Could you check a few things on this model? Use its own coordinates, in mm. Face numbers are marked on the shaded views. A direction names the side the tool comes from. Coordinates: 2 decimals unless noted, no trailing zeros.
```python
from build123d import *

# Parameters (mm, degrees)
SKETCH1_RX          = 12
SKETCH1_RY          = 6.5
SKETCH1_R           = 1.1
BOSS_EXTRUDE1_DEPTH = 1
SKETCH2_R           = 6.5
BOSS_EXTRUDE2_DEPTH = 2
SKETCH4_R           = 5.5
BOSS_EXTRUDE3_DEPTH = 7
BOSS_EXTRUDE5_START = 0.25
SKETCH7_R           = 5.5
BOSS_EXTRUDE5_DEPTH = 0.25
SKETCH5_R           = 0.75
CUT_EXTRUDE2_DEPTH  = 7
SKETCH6_R           = 0.75
BOSS_EXTRUDE4_DEPTH = 3.4
FILLET1_R           = 0.25


with BuildPart() as part:
    # Sketch1 → Boss-Extrude1 (new body)
    with BuildSketch(Plane(origin=(0, 0, 0), x_dir=(1, 0, 0), z_dir=(0, 1, 0))):
        with Locations(Location((0, 0), (0, 0, 180))):
            Ellipse(SKETCH1_RX, SKETCH1_RY)
        with Locations(Location((-9, 0, 0), (0, 0, 270))):
            Circle(SKETCH1_R, mode=Mode.SUBTRACT)
        with Locations(Location((9, 0, 0), (0, 0, 270))):
            Circle(SKETCH1_R, mode=Mode.SUBTRACT)
    extrude(amount=BOSS_EXTRUDE1_DEPTH)

    # Sketch2 → Boss-Extrude2 (add)
    with BuildSketch(Plane(origin=(0, 1, 0), x_dir=(1, 0, 0), z_dir=(0, 1, 0))):
        with Locations(Location((0, 0, 0), (0, 0, 270))):
            Circle(SKETCH2_R)
    extrude(amount=BOSS_EXTRUDE2_DEPTH)

    # Sketch4 → Boss-Extrude3 (add)
    with BuildSketch(Plane.XZ):
        with Locations(Location((0, 0, 0), (0, 0, 90))):
            Circle(SKETCH4_R)
    extrude(amount=BOSS_EXTRUDE3_DEPTH)

    # Sketch7 → Boss-Extrude5 (add)
    with BuildSketch(Plane(origin=(0, 3, 0), x_dir=(1, 0, 0), z_dir=(0, 1, 0)).offset(BOSS_EXTRUDE5_START)):
        with Locations(Location((0, 0, 0), (0, 0, 270))):
            Circle(SKETCH7_R)
    extrude(amount=-BOSS_EXTRUDE5_DEPTH)

    # Sketch5 → Cut-Extrude2 (cut)
    with BuildSketch(Plane(origin=(0, 3.25, 0), x_dir=(1, 0, 0), z_dir=(0, 1, 0))):
        with Locations(Location((0, -4, 0), (0, 0, 270))):
            Circle(SKETCH5_R)
        with Locations(Location((-1.735534956, -3.603875472, 0), (0, 0, 270))):
            Circle(SKETCH5_R)
        with Locations(Location((-3.12732593, -2.493959207, 0), (0, 0, 270))):
            Circle(SKETCH5_R)
        with Locations(Location((-3.899711649, -0.890083736, 0), (0, 0, 270))):
            Circle(SKETCH5_R)
        with Locations(Location((-3.899711649, 0.890083736, 0), (0, 0, 270))):
            Circle(SKETCH5_R)
        with Locations(Location((-3.12732593, 2.493959207, 0), (0, 0, 270))):
            Circle(SKETCH5_R)
        with Locations(Location((-1.735534956, 3.603875472, 0), (0, 0, 270))):
            Circle(SKETCH5_R)
        with Locations(Location((0, 4, 0), (0, 0, 270))):
            Circle(SKETCH5_R)
        with Locations(Location((1.735534956, 3.603875472, 0), (0, 0, 270))):
            Circle(SKETCH5_R)
        with Locations(Location((3.12732593, 2.493959207, 0), (0, 0, 270))):
            Circle(SKETCH5_R)
        with Locations(Location((3.899711649, 0.890083736, 0), (0, 0, 270))):
            Circle(SKETCH5_R)
        with Locations(Location((3.899711649, -0.890083736, 0), (0, 0, 270))):
            Circle(SKETCH5_R)
        with Locations(Location((3.12732593, -2.493959207, 0), (0, 0, 270))):
            Circle(SKETCH5_R)
        with Locations(Location((1.735534956, -3.603875472, 0), (0, 0, 270))):
            Circle(SKETCH5_R)
    extrude(amount=-CUT_EXTRUDE2_DEPTH, mode=Mode.SUBTRACT)

    # Sketch6 → Boss-Extrude4 (add)
    with BuildSketch(Plane.XZ.offset(7)):
        with Locations(Location((0, -4, 0), (0, 0, 90))):
            Circle(SKETCH6_R)
        with Locations(Location((-1.735534956, -3.603875472, 0), (0, 0, 90))):
            Circle(SKETCH6_R)
        with Locations(Location((-3.12732593, -2.493959207, 0), (0, 0, 90))):
            Circle(SKETCH6_R)
        with Locations(Location((-3.899711649, -0.890083736, 0), (0, 0, 90))):
            Circle(SKETCH6_R)
        with Locations(Location((-3.899711649, 0.890083736, 0), (0, 0, 90))):
            Circle(SKETCH6_R)
        with Locations(Location((-3.12732593, 2.493959207, 0), (0, 0, 90))):
            Circle(SKETCH6_R)
        with Locations(Location((-1.735534956, 3.603875472, 0), (0, 0, 90))):
            Circle(SKETCH6_R)
        with Locations(Location((0, 4, 0), (0, 0, 90))):
            Circle(SKETCH6_R)
        with Locations(Location((1.735534956, 3.603875472, 0), (0, 0, 90))):
            Circle(SKETCH6_R)
        with Locations(Location((3.12732593, 2.493959207, 0), (0, 0, 90))):
            Circle(SKETCH6_R)
        with Locations(Location((3.899711649, 0.890083736, 0), (0, 0, 90))):
            Circle(SKETCH6_R)
        with Locations(Location((3.899711649, -0.890083736, 0), (0, 0, 90))):
            Circle(SKETCH6_R)
        with Locations(Location((3.12732593, -2.493959207, 0), (0, 0, 90))):
            Circle(SKETCH6_R)
        with Locations(Location((1.735534956, -3.603875472, 0), (0, 0, 90))):
            Circle(SKETCH6_R)
    extrude(amount=BOSS_EXTRUDE4_DEPTH)

    # Fillet1
    fillet1_edges = [part.edges().sort_by_distance(p)[0] for p in [
        (0, 3, -5.5),
    ]]
    fillet(fillet1_edges, radius=FILLET1_R - 0.0001)  # a hair under: the kernel refuses the full size


solid = part.part
```
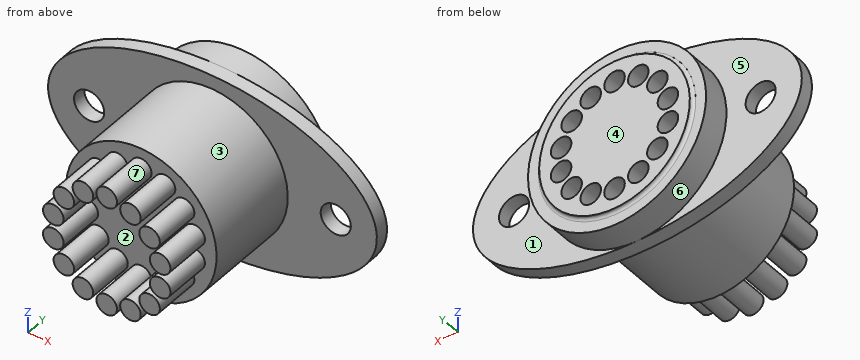
1. On a 3-axis mill with a long thin cutter (end or side, diameter ignored), from which of +Z, -Z, +X, -X, +Y, -Y can I reach the whole of each face in a straight line? I mean the marked faces 4, 5, 6 and 7. Say none if no direction works.
Verdict:
face 4: +Z, -Z, +X, -X, +Y
face 5: -X, +Y
face 6: +Y
face 7: -Y
2. I want a section at A-A on y = -9.25. Give the number of separate pieces and of enclosed holes in the cut face, plus the area to 3 significant figures.
Verdict:
separate pieces: 14
enclosed holes: 0
area: 24.7 mm2
3. For pin 1 (1 mm diameter, centred on y = 0, z = -3.5, fed in from -X); pin 2 (1.4 mm diameter, centred on x = -3.9, z = -0.89, fed in from +Y); pin 3 (1.6 mm diameter, centred on x = 4, z = 1, fed in from +Y); pin 4 (3 mm diameter, centred on x = -7.5, z = 1, fed in from -Y), each with a flat end and sliding along its axis, tell me the tip position at first contact or that it passes through.
Verdict:
pin 1: stops at x = -10.65
pin 2: stops at y = -3.75
pin 3: stops at y = 3.25
pin 4: stops at y = 0
4. Please list where these lines run through material, in increasing order: line 1 along X through (y, z) = (0.5, 0); line 2 along X through (y, z) = (-0.5, 3.75); line 3 along X through (y, z) = (0.5, 4).
Verdict:
line 1: x = -12 to -10.1, -7.9 to 7.9, 10.1 to 12
line 2: x = -4.02 to -2.47, -1 to -0.71, 0.71 to 1, 2.47 to 4.02
line 3: x = -9.46 to -2.37, -1.1 to -0.75, 0.75 to 1.1, 2.37 to 9.46
5. If we mould it in two halves opening along Z, with no side actions, what happens to the marked faces 1, 2 and 3? For each: pulls with the +Z half, pulls with the -Z half, needs draft (parallel to the pull), parting line crosses it, or undercut.
Verdict:
face 1: needs draft
face 2: undercut
face 3: parting line crosses it
